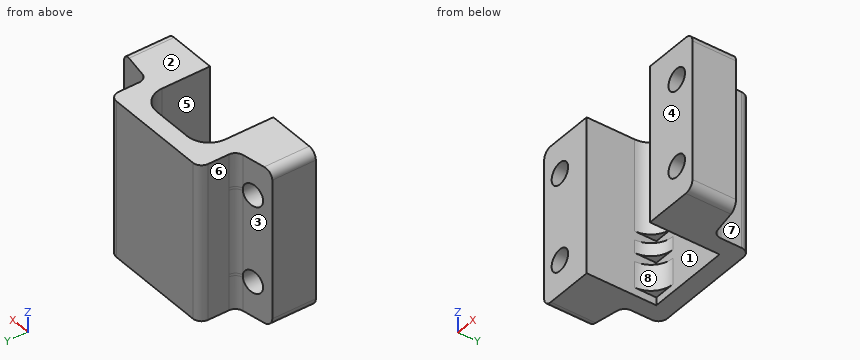
from build123d import *

# Parameters (mm, degrees)
BOSS_EXTRUDE1_DEPTH = 22.86
BOSS_EXTRUDE2_DEPTH = 13.462
BOSS_EXTRUDE3_START = -1.27
BOSS_EXTRUDE3_DEPTH = 1.905
BOSS_EXTRUDE4_START = -1.27
BOSS_EXTRUDE4_DEPTH = 3.81
FILLET1_R           = 1.27


with BuildPart() as part:
    # Sketch1 → Boss-Extrude1 (new body)
    with BuildSketch(Plane.XY):
        Polygon((-6.096, 10.16), (6.096, 10.16), (6.096, 0), (14.2875, 0), (14.2875, 6.35), (8.636, 7.346511931), (8.636, 12.7), (-8.636, 12.7), (-8.636, 7.346511931), (-14.2875, 6.35), (-14.2875, 0), (-6.096, 0), align=None)
    extrude(amount=-BOSS_EXTRUDE1_DEPTH)

    # Sketch2 → Boss-Extrude2 (add)
    with BuildSketch(Plane.XY):
        with BuildLine():
            Line((2.921, 10.16), (6.096, 10.16))
            Line((6.096, 10.16), (6.096, 6.985))
            ThreePointArc((6.096, 6.985), (5.16606403, 9.23006403), (2.921, 10.16))
        make_face()
        with BuildLine():
            Line((-6.096, 10.16), (-6.096, 6.985))
            ThreePointArc((-6.096, 6.985), (-5.16606403, 9.23006403), (-2.921, 10.16))
            Line((-2.921, 10.16), (-6.096, 10.16))
        make_face()
    extrude(amount=-BOSS_EXTRUDE2_DEPTH)

    # Sketch3 → Boss-Extrude3 (add)
    with BuildSketch(Plane.XY.offset(-13.462).offset(BOSS_EXTRUDE3_START)):
        with BuildLine():
            Line((-6.096, 10.16), (-6.096, 6.985))
            ThreePointArc((-6.096, 6.985), (-5.16606403, 9.23006403), (-2.921, 10.16))
            Line((-2.921, 10.16), (-6.096, 10.16))
        make_face()
    extrude(amount=-BOSS_EXTRUDE3_DEPTH)

    # Sketch4 → Boss-Extrude4 (add)
    with BuildSketch(Plane.XY.offset(-16.637).offset(BOSS_EXTRUDE4_START)):
        with BuildLine():
            Line((-6.096, 10.16), (-6.096, 6.985))
            ThreePointArc((-6.096, 6.985), (-5.16606403, 9.23006403), (-2.921, 10.16))
            Line((-2.921, 10.16), (-6.096, 10.16))
        make_face()
    extrude(amount=-BOSS_EXTRUDE4_DEPTH)

    # Sketch6 → Cut-Revolve1 (revolve, cut)
    with BuildSketch(Plane.XY.offset(-5.08)):
        Polygon((11.262482277, -1.27), (12.849982277, -1.27), (12.849982277, 6.60347316), (12.849982277, 9.423392242), (11.262482277, 9.423392242), (11.262482277, 6.883392242), align=None)
    cut_revolve1 = revolve(axis=Axis((11.262482277, -1.27, -5.08), (0, -1, 0)), mode=Mode.SUBTRACT)

    # Mirror1: Cut-Revolve1 across plane
    add(cut_revolve1.mirror(Plane(origin=(0, 0, 0), x_dir=(0, 0, 1), z_dir=(1, 0, 0))), mode=Mode.SUBTRACT)

    # Mirror2: Cut-Revolve1 across plane
    add(cut_revolve1.mirror(Plane.XY.offset(-11.43)), mode=Mode.SUBTRACT)

    # Mirror2 copy 1 sketch → Mirror2 copy 1 (revolve, cut)
    with BuildSketch(Plane(origin=(0, 0, -17.78), x_dir=(-1, 0, 0), z_dir=(0, 0, -1))):
        Polygon((11.262482277, -1.27), (12.849982277, -1.27), (12.849982277, 6.60347316), (12.849982277, 9.423392242), (11.262482277, 9.423392242), (11.262482277, 6.883392242), align=None)
    revolve(axis=Axis((-11.262482277, -1.27, -17.78), (0, -1, 0)), mode=Mode.SUBTRACT)

    # Fillet1
    fillet1_edges = [part.edges().sort_by_distance(p)[0] for p in [
        (-14.2875, 3.175, 0),
        (14.2875, 3.175, 0),
        (14.2875, 3.175, -22.86),
        (-8.636, 7.346511931, -11.43),
        (-8.636, 12.7, -11.43),
        (8.636, 12.7, -11.43),
        (8.636, 7.346511931, -11.43),
        (-14.2875, 3.175, -22.86),
    ]]
    fillet(fillet1_edges, radius=FILLET1_R)


solid = part.part
Input: part model. Units: mm. Frame: model coordinates. Face numbers are marked on the shaded views. A direction names the side the tool comes from. Coordinates: 2 decimals unless noted, no trailing zeros. Order: outer loops, then holes, each group sorted by start corner. A loop starts at its lowest first (then second) coordinate and runs counter-clockwise, first axis right, second up. Notation, with made-up numbers: M 71.25,50 L 100.25,50 A17 cw 100.25,72 Z; hole C -20.75,75 d1. An arc over 180 degrees is marked long. Answer in a Markdown table with one row per item.
(1) Access query for the marked faces 4, 5, 6, 7 and 8. Directions: +Z, -Z, +X, -X, +Y, -Y. A direction counts if a zero-diameter tool reaches every point of the face in a straight line with its end or side. Return the directions, or none.
Numbers:
| item | result |
|---|---|
| face 4 | +Z, -Z, +X, -X, -Y |
| face 5 | -Z, -Y |
| face 6 | +Z, -Z, -X, +Y |
| face 7 | +Z, -Z, +X, +Y |
| face 8 | +Z, -Z, -Y |
(2) Contact query for flat-ended pins moving along their axis: pin 1 Ø3.5 at (x, z) = (11.26, -17.78) entering from +Y; pin 2 Ø10 at (x, z) = (-9.5, -15) entering from +Y; pin 3 Ø1.5 at (y, z) = (10, -6.5) entering from +X; pin 4 Ø6 at (x, z) = (-1.5, -10.5) entering from -Y. Output: stop coordinate, or through.
Numbers:
| item | result |
|---|---|
| pin 1 | stops at y = 7.21 |
| pin 2 | stops at y = 12.7 |
| pin 3 | stops at x = 8.64 |
| pin 4 | stops at y = 9.74 |
(3) Section query C-C, the plane x = 10.5. Output: boundary loops of the cut face in (y, z), plus the area to 3 significant figures.
Numbers:
| item | result |
|---|---|
| outline | M 0,-22.86 L 7.02,-22.86 L 7.02,-19.17 L 0,-19.17 Z; M 0,-16.39 L 7.02,-16.39 L 7.02,-6.47 L 0,-6.47 Z; M 0,-3.69 L 7.02,-3.69 L 7.02,0 L 0,0 Z |
| area | 121 mm^2 |
(4) Section query D-D, the plane y = 8.75. Output: boundary loops of the cut face in (x, z).
Numbers:
| item | result |
|---|---|
| outline | M -8.64,-22.86 L -6.1,-22.86 L -6.1,-21.72 L -5.56,-21.72 L -5.56,-17.91 L -6.1,-17.91 L -6.1,-16.64 L -5.56,-16.64 L -5.56,-14.73 L -6.1,-14.73 L -6.1,-13.46 L -5.56,-13.46 L -5.56,0 L -8.64,0 Z; M 5.56,-13.46 L 6.1,-13.46 L 6.1,-22.86 L 8.64,-22.86 L 8.64,0 L 5.56,0 Z |
(5) Draft query along X for the marked faces 1, 2 and 3. Return one class per face: pulls with the +X half, pulls with the -X half, needs draft (parallel to the pull), parting line crosses it, or undercut.
Numbers:
| item | result |
|---|---|
| face 1 | undercut |
| face 2 | needs draft |
| face 3 | pulls with the -X half |
(6) Material intervals for line 1 (X direction, y = 1.5, z = -17.78); line 2 (X direction, y = 5.75, z = -7.25); line 3 (X direction, y = 5.75, z = -6.5), sorted ascending. Write a range as [from, to].
Numbers:
| item | result |
|---|---|
| line 1 | x = [-14.29, -12.85], [-9.67, -6.1], [6.1, 9.67], [12.85, 14.29] |
| line 2 | x = [-14.29, -6.1], [6.1, 14.29] |
| line 3 | x = [-14.29, -11.97], [-10.55, -6.1], [6.1, 10.55], [11.97, 14.29] |
(7) Section query A-A, the plane y = 5.5. Output: boundary loops of the cut face in (x, z) (1 decimal).
Numbers:
| item | result |
|---|---|
| outline | M -14.3,-21.6 A1.3 ccw -13,-22.9 L -6.1,-22.9 L -6.1,0 L -13,0 A1.3 ccw -14.3,-1.3 Z; M 6.1,-22.9 L 13,-22.9 A1.3 ccw 14.3,-21.6 L 14.3,-1.3 A1.3 ccw 13,0 L 6.1,0 Z; hole C -11.3,-17.8 d3.2; hole C -11.3,-5.1 d3.2; hole C 11.3,-17.8 d3.2; hole C 11.3,-5.1 d3.2 |
